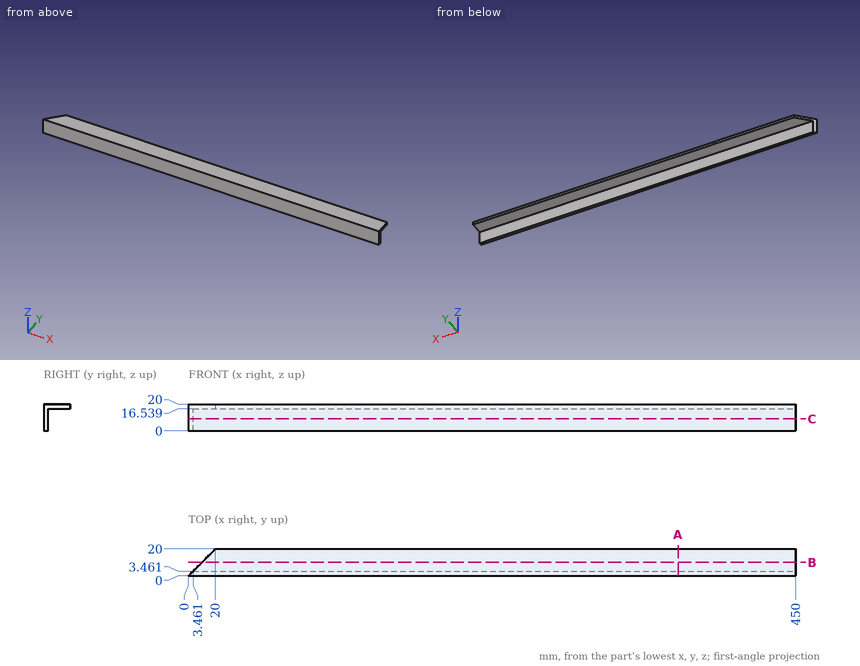
Print and shaded views of the part. All mm, measured from the part's lowest x, y and z. Coordinates: 2 decimals unless noted, no trailing zeros. Loops run counter-clockwise (first coordinate to the right, second up) from the corner with the lowest first, then second, coordinate; pieces in that order, holes last. Notation, with made-up numbers: (-9, -32.5) -> (42, -32.5) arc R24 cw to (42, 5.5) -> close; hole circle Ø5 at (6.25, -14). An arc over 180 degrees is marked (long way). Use a Markdown table: item, result. Add a question column.
Item 1: Probe probe 1 along Y at (x, z) = (34.5, 12.5); probe 2 along Z at (x, y) = (398.5, 8); probe 3 along X at (y, z) = (14.25, 17.5). List the from-to ranges inside material, lowest first.
Item 2: Band-saw the part on A-A on x = 363. Write the cut outline in (y, z).
Item 3: Band-saw the part on B-B on y = 10. Write the cut outline in (x, z).
Item 4: Flat gauge pins, fed straight in: P1, Ø1.5, axis at x = 106, z = 9, coming from the +Y side; P2, Ø8, axis at x = 298, y = 10, coming from the -Z side. Where does each tip first touch, or does it go through?
Item 5: Band-saw the part on C-C on z = 9. Write the cut outline in (x, y), plus the area to 3 significant figures.
Geometry says:
| question | item | result |
|---|---|---|
| 1 | probe 1 | 0 to 3.46 |
| 1 | probe 2 | 16.54 to 20 |
| 1 | probe 3 | 14.25 to 450 |
| 2 | outline | (0, 0) -> (3.46, 0) -> (3.46, 16.54) -> (20, 16.54) -> (20, 20) -> (0, 20) -> close |
| 3 | outline | (10, 16.54) -> (450, 16.54) -> (450, 20) -> (10, 20) -> close |
| 4 | P1 | y = 3.46 |
| 4 | P2 | z = 16.54 |
| 5 | outline | (0, 0) -> (450, 0) -> (450, 3.46) -> (3.46, 3.46) -> close |
| 5 | area | 1,550 mm² |
